```python
from build123d import *

# Parameters (mm, degrees)
SKETCH1_W           = 35
SKETCH1_H           = 30
BOSS_EXTRUDE1_DEPTH = 28
SKETCH2_R           = 1.5
CUT_EXTRUDE1_DEPTH  = 10
SKETCH3_R           = 11
CUT_EXTRUDE2_DEPTH  = 5
SKETCH4_R           = 5
CUT_EXTRUDE3_DEPTH  = 42.41557678


with BuildPart() as part:
    # Sketch1 → Boss-Extrude1 (new body)
    with BuildSketch(Plane(origin=(0, 0, 0), x_dir=(1, 0, 0), z_dir=(0, 1, 0))):
        Rectangle(SKETCH1_W, SKETCH1_H)
    extrude(amount=BOSS_EXTRUDE1_DEPTH)

    # Sketch2 → Cut-Extrude1 (cut)
    with BuildSketch(Plane.XY.offset(15)):
        with Locations((-12.5, 23)):
            Circle(SKETCH2_R)
        with Locations((12.5, 23)):
            Circle(SKETCH2_R)
        with Locations((12.5, 5)):
            Circle(SKETCH2_R)
        with Locations((-12.5, 5)):
            Circle(SKETCH2_R)
    extrude(amount=-CUT_EXTRUDE1_DEPTH, mode=Mode.SUBTRACT)

    # Sketch3 → Cut-Extrude2 (cut)
    with BuildSketch(Plane(origin=(0, 0, -15), x_dir=(-1, 0, 0), z_dir=(0, 0, -1))):
        with Locations((0, 14)):
            Circle(SKETCH3_R)
    extrude(amount=-CUT_EXTRUDE2_DEPTH, mode=Mode.SUBTRACT)

    # Sketch4 → Cut-Extrude3 (cut, through all)
    with BuildSketch(Plane(origin=(0, 0, -10), x_dir=(-1, 0, 0), z_dir=(0, 0, -1))):
        with Locations((0, 14)):
            Circle(SKETCH4_R)
    extrude(amount=-CUT_EXTRUDE3_DEPTH, mode=Mode.SUBTRACT)


solid = part.part
```
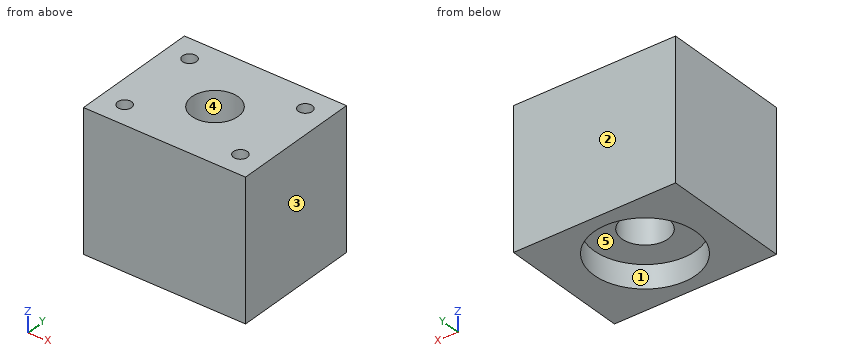
Read the model definition and answer for the solid it produces. Units are mm, in the model's axes. Face numbers are marked on the shaded views. A direction names the side the tool comes from. Coordinates: 2 decimals unless noted, no trailing zeros. Loops run counter-clockwise (first coordinate to the right, second up) from the corner with the lowest first, then second, coordinate; pieces in that order, holes last.
(1) The part is cut by section A-A (x = 0). Determine the outline of the cut face in (y, z).
Solution:
outline: (0, -15) - (3, -15) - (3, -10) - (9, -10) - (9, 15) - (0, 15) - close; (19, -10) - (25, -10) - (25, -15) - (28, -15) - (28, 15) - (19, 15) - close
(2) The part is cut by section C-C (z = -0.25). Determine the outline of the cut face in (x, y).
Solution:
outline: (-17.5, 0) - (17.5, 0) - (17.5, 28) - (-17.5, 28) - close; hole circle Ø10 at (0, 14)
(3) Consider line 1 along Y through (x, z) = (-12.5, 7.5); line 2 along Y through (x, z) = (0, -0.5); line 3 along Y through (x, z) = (0, -12.9). Determine where each line is inside the solid, lowest interval first.
Solution:
line 1: y = 0 to 3.5, 6.5 to 21.5, 24.5 to 28
line 2: y = 0 to 9, 19 to 28
line 3: y = 0 to 3, 25 to 28
(4) The mould has two halves that part along X. Classify the marked faces 1, 2 and 3: released by +X, released by -X, zero draft, split by the parting line, or undercut.
Solution:
face 1: undercut
face 2: zero draft
face 3: released by +X
(5) The part is cut by section D-D (z = 8). Determine the outline of the cut face in (x, y).
Solution:
outline: (-17.5, 0) - (17.5, 0) - (17.5, 28) - (-17.5, 28) - close; hole circle Ø3 at (-12.5, 5); hole circle Ø3 at (-12.5, 23); hole circle Ø10 at (0, 14); hole circle Ø3 at (12.5, 5); hole circle Ø3 at (12.5, 23)
(6) A tool of negligible diameter and unlimited length cuts with its end or side. For the marked faces 4 and 5, from which of +Z, -Z, +X, -X, +Y, -Y can it reach the whole face along a straight path? Write none if from no direction.
Solution:
face 4: +Z, -Z
face 5: -Z
(7) The part is cut by section B-B (y = 14). Determine the outline of the cut face in (x, z).
Solution:
outline: (-17.5, -15) - (-11, -15) - (-11, -10) - (-5, -10) - (-5, 15) - (-17.5, 15) - close; (5, -10) - (11, -10) - (11, -15) - (17.5, -15) - (17.5, 15) - (5, 15) - close
(8) Flat-ended cylindrical pins translate along their axes: pin 1 Ø1.5 at (x, y) = (13, 22.5) entering from +Z; pin 2 Ø8 at (x, y) = (0, 14) entering from +Z. Find the tip coordinate at first contact, or state that the pin passes through.
Solution:
pin 1: stops at z = 5
pin 2: passes through
